Design review of the part built by this model. Coordinates are the model's own, in mm. A direction names the side the tool comes from. Round coordinates to 2 decimals unless told otherwise and drop trailing zeros. Write each loop counter-clockwise with the first axis right and the second up, starting at its lowest first coordinate (ties: lowest second). Pieces come first, ordered by that corner, then holes.
from build123d import *

# Parameters (mm, degrees)
F0_W      = 31.75
F0_H      = 31.75
F1_DEPTH  = 6.35
F2_W      = 6.35
F2_H      = 31.75
F3_DEPTH  = 10.16
F4_W      = 6.35
F4_H      = 31.75
F5_DEPTH  = 10.16
F6_W      = 12.7
F6_H      = 38.1
F7_DEPTH  = 12.7
F8_W      = 3.175
F8_H      = 6.35
F9_DEPTH  = 12.7
F10_W     = 12.7
F10_H     = 19.05
F11_DEPTH = 12.7
F13_W     = 10.16
F13_H     = 1.27
F14_DEPTH = 4.7625
F16_DEPTH = 19.05
F17_W     = 3.175
F17_H     = 1.27
F18_DEPTH = 4.7498


with BuildPart() as f1:
    # F0 (on Front) → F1 (new body)
    with BuildSketch(Plane.XZ):
        with Locations((15.875, 15.875)):
            Rectangle(F0_W, F0_H)
    extrude(amount=F1_DEPTH)

    # F2 (on face) → F3 (join)
    with BuildSketch(Plane(origin=(0, 0, 0), x_dir=(0, -1, 0), z_dir=(-1, 0, 0))):
        Polygon((0, 0), (0, -25.4), (25.4, -25.4), (25.4, 31.75), (6.35, 31.75), (6.35, 0), align=None)
        with Locations((3.175, 15.875)):
            Rectangle(F2_W, F2_H)
    extrude(amount=F3_DEPTH)

    # F4 (on face) → F5 (join)
    with BuildSketch(Plane.YZ.offset(31.75)):
        with Locations((-3.175, 15.875)):
            Rectangle(F4_W, F4_H)
        Polygon((-6.35, 0), (-6.35, 31.75), (-25.4, 31.75), (-25.4, -25.4), (0, -25.4), (0, 0), align=None)
    extrude(amount=F5_DEPTH)

    # F6 (on face) → F7 (cut)
    with BuildSketch(Plane.YZ.offset(41.91)):
        with Locations((-12.7, -6.35)):
            Rectangle(F6_W, F6_H)
    extrude(amount=-F7_DEPTH, mode=Mode.SUBTRACT)

    # F8 (on face) → F9 (join, through all)
    with BuildSketch(Plane.XZ.offset(6.35)):
        with Locations((40.3225, -3.175)):
            Rectangle(F8_W, F8_H)
    extrude(amount=F9_DEPTH)

    # F10 (on face) → F11 (cut)
    with BuildSketch(Plane(origin=(-10.16, 0, 0), x_dir=(0, -1, 0), z_dir=(-1, 0, 0))):
        with Locations((12.7, -15.875)):
            Rectangle(F10_W, F10_H)
    extrude(amount=-F11_DEPTH, mode=Mode.SUBTRACT)

    # F13 (on face) → F14 (join)
    with BuildSketch(Plane(origin=(0, 0, -6.35), x_dir=(1, 0, 0), z_dir=(0, 0, -1))):
        with Locations((-5.08, 12.7)):
            Rectangle(F13_W, F13_H)
    extrude(amount=F14_DEPTH)

    # F15 (on face) → F16 (join)
    with BuildSketch(Plane.XZ.offset(6.35)):
        with BuildLine():
            Line((16.4158089086, 15.6251635376), (15.875, 15.875))
            Line((15.875, 15.875), (19.2451557873, 21.9931921324))
            ThreePointArc((19.2451557873, 21.9931921324), (12.2474155401, 9.9058412664), (19.7534345525, 21.6843003384))
            Line((19.7534345525, 21.6843003384), (16.4158089086, 15.6251635376))
        make_face()
    extrude(amount=F16_DEPTH)

    # F17 (on face) → F18 (join)
    with BuildSketch(Plane(origin=(0, 0, -6.35), x_dir=(1, 0, 0), z_dir=(0, 0, -1))):
        with Locations((40.3225, 12.7)):
            Rectangle(F17_W, F17_H)
    extrude(amount=F18_DEPTH)


solid = f1.part
1) Add section B-B on y = -9.25. State the section outline as (x, z) points (3 decimals), and give its area (3 significant figures).
2) For P1, Ø12, axis at x = 30, z = -6, coming from the -Y side; P2, Ø1, axis at x = -6, y = -13, coming from the -Z side; P3, Ø1.6, axis at x = 40.5, y = -9.5, coming from the -Z side; P4, Ø7, axis at x = 8.5, y = -3.5, coming from the -Z side, all flat-tipped, find the tip position at first contact; note any pin that passes through.
3) Add section A-A on z = -14.5. State the section outline as (x, y) points.
4) The part is to be moulded in two halves that separate along X. For faces 4 (the face through (-10.16, -13, 10)), 5 (the face through (17.536, -15.742, 18.891)), 6 (the face through (37, -3, -25.4)), say which applies: pulls with the +X half, pulls with the -X half, needs draft (parallel to the pull), parting line crosses it, or undercut.
5) For line 1 along X through (y, z) = (-24, -4); line 2 along Y through (x, z) = (-7, -23); line 3 along X through (y, z) = (-8.25, 14.5), list the stretches that pass through material, from the lowest coordinate up.
6) Add section C-C on y = -21.5. State the section outline as (x, z) points (3 decimals).
7) Add section D-D on z = -4. State the section outline as (x, y) points (3 decimals).
8) For faces 1 (the face through (31.75, -3, -13)), 2 (the face through (18.11, -15.74, 18.7)), 3 (the face through (-5, -9, -6.35)), list the 3-axis set-ups (+Z, -Z, +X, -X, +Y, -Y) from which the entire face can be reached by the end or side of a thin tool; tool diameter is ignored.
Computed:
1. outline: (-10.16, -6.35) - (0, -6.35) - (0, 31.75) - (-10.16, 31.75) - close; (15.875, 15.875) - (19.245, 21.993) arc R6.985 ccw (long way) to (19.753, 21.684) - (16.416, 15.625) - close; (31.75, 12.7) - (41.91, 12.7) - (41.91, 31.75) - (31.75, 31.75) - close; (38.735, -6.35) - (41.91, -6.35) - (41.91, 0) - (38.735, 0) - close
1. area: 750 mm2
2. P1: stops at y = -25.4
2. P2: stops at z = -11.11
2. P3: stops at z = -6.35
2. P4: stops at z = 0
3. outline: (-10.16, -25.4) - (0, -25.4) - (0, -19.05) - (-10.16, -19.05) - close; (-10.16, -6.35) - (0, -6.35) - (0, 0) - (-10.16, 0) - close; (31.75, -25.4) - (41.91, -25.4) - (41.91, -19.05) - (31.75, -19.05) - close; (31.75, -6.35) - (41.91, -6.35) - (41.91, 0) - (31.75, 0) - close
4. face 4: pulls with the -X half
4. face 5: undercut
4. face 6: needs draft
5. line 1: x = -10.16 to 0, 31.75 to 41.91
5. line 2: y = -25.4 to -19.05, -6.35 to 0
5. line 3: x = -10.16 to 0, 9.03 to 22.72, 31.75 to 41.91
6. outline: (-10.16, -25.4) - (0, -25.4) - (0, 31.75) - (-10.16, 31.75) - close; (15.875, 15.875) - (19.245, 21.993) arc R6.985 ccw (long way) to (19.753, 21.684) - (16.416, 15.625) - close; (31.75, -25.4) - (41.91, -25.4) - (41.91, 31.75) - (31.75, 31.75) - close
7. outline: (-10.16, -25.4) - (0, -25.4) - (0, 0) - (-10.16, 0) - close; (31.75, -25.4) - (41.91, -25.4) - (41.91, 0) - (31.75, 0) - (31.75, -6.35) - (38.735, -6.35) - (38.735, -19.05) - (31.75, -19.05) - close
8. face 1: -Z, +Y, -Y
8. face 2: -Y
8. face 3: -Z, +X, -X
